CAD build for the part. Positions are in the model's coordinates, mm. A direction names the side the tool comes from. Give positions to 0.01 mm unless a question says otherwise; leave off trailing zeros. Write each loop counter-clockwise with the first axis right and the second up, starting at its lowest first coordinate (ties: lowest second). Pieces come first, ordered by that corner, then holes. Notation, with made-up numbers: (57.5, 22) -> (102.5, 22) arc R25 cw to (102.5, 56) -> close; hole circle Ø7 at (-34.75, 84). An arc over 180 degrees is marked (long way). Answer as a JSON object with one key per item and string values.
```python
from build123d import *

# Parameters (mm, degrees)
F0_W           = 11.5
F0_H           = 30
F1_DEPTH       = 1.5
F2_D           = 2.5
F2_CSINK_D     = 5
F2_CSINK_ANGLE = 90
F4_DEPTH       = 25
F5_R           = 1.49999


# Not quite as in the source:
# - a fillet or chamfer is up to 0.001 mm smaller than in the source, because OpenCascade refuses the exact size


with BuildPart() as f1:
    # F0 (on Front) → F1 (new body)
    with BuildSketch(Plane.XZ):
        with BuildLine():
            ThreePointArc((-3.8116748205, 37.8448306397), (-9.5616748205, 43.5948306397), (-15.3116748205, 37.8448306397))
            Line((-15.3116748205, 37.8448306397), (-3.8116748205, 37.8448306397))
        make_face()
        with Locations((-9.5616748205, 22.8448306397)):
            Rectangle(F0_W, F0_H)
        with BuildLine():
            Line((-3.8116748205, 7.8448306397), (-15.3116748205, 7.8448306397))
            ThreePointArc((-15.3116748205, 7.8448306397), (-9.5616748205, 2.0948306397), (-3.8116748205, 7.8448306397))
        make_face()
    extrude(amount=F1_DEPTH)

    # F2 (through all)
    with Locations(Plane(origin=(0, 0, 0), x_dir=(1, 0, 0), z_dir=(0, 1, 0))):
        with Locations((-9.5616748205, -37.8448306397), (-9.5616748205, -7.8448306397)):
            CounterSinkHole(F2_D / 2, F2_CSINK_D / 2, counter_sink_angle=F2_CSINK_ANGLE)

    # F3 (on face) → F4 (cut)
    with BuildSketch(Plane.XZ):
        with BuildLine():
            Line((-8.1408721001, 19.8448306397), (-8.1408721001, 25.8448306397))
            Line((-8.1408721001, 25.8448306397), (-11.1408721001, 25.8448306397))
            Line((-11.1408721001, 25.8448306397), (-11.1408721001, 19.8448306397))
            ThreePointArc((-11.1408721001, 19.8448306397), (-9.6408721001, 20.3448306397), (-8.1408721001, 19.8448306397))
        make_face()
        with BuildLine():
            ThreePointArc((-7.1408721001, 17.8448306397), (-7.4048041226, 18.9628646284), (-8.1408721001, 19.8448306397))
            Line((-8.1408721001, 19.8448306397), (-8.1408721001, 17.8448306397))
            Line((-8.1408721001, 17.8448306397), (-11.1408721001, 17.8448306397))
            Line((-11.1408721001, 17.8448306397), (-11.1408721001, 19.8448306397))
            ThreePointArc((-11.1408721001, 19.8448306397), (-10.7589060888, 15.6087626622), (-7.1408721001, 17.8448306397))
        make_face()
        with BuildLine():
            Line((-8.1408721001, 17.8448306397), (-8.1408721001, 19.8448306397))
            ThreePointArc((-8.1408721001, 19.8448306397), (-9.6408721001, 20.3448306397), (-11.1408721001, 19.8448306397))
            Line((-11.1408721001, 19.8448306397), (-11.1408721001, 17.8448306397))
            Line((-11.1408721001, 17.8448306397), (-8.1408721001, 17.8448306397))
        make_face()
    extrude(amount=F4_DEPTH, mode=Mode.SUBTRACT)

    # F5 (radius 1.5 in the source; OpenCascade refuses exactly that, so slightly less here)
    f5_edges = [f1.edges().sort_by_distance(p)[0] for p in [
        (-8.140872, -0.75, 25.844831),
        (-11.140872, -0.75, 25.844831),
    ]]
    fillet(f5_edges, radius=F5_R)


solid = f1.part
```
1) Slice it at C-C (x = -6). List the corners of the cut face in (y, z), then the cut area to 3 significant figures.
Model answer:
{"outline": "(-1.5, 3.33) -> (0, 3.33) -> (0, 42.36) -> (-1.5, 42.36) -> close", "area": "58.5 mm2"}
2) Slice it at A-A (y = -0.35). State how many separate pieces and enclosed holes the cut face has, then the cut area to 3 significant figures.
Model answer:
{"separate pieces": "1", "enclosed holes": "3", "area": "384 mm2"}
3) Slice it at B-B (z = 17.5). List the corners of the cut face in (x, y), then the cut area to 3 significant figures.
Model answer:
{"outline": "(-15.31, -1.5) -> (-12.12, -1.5) -> (-12.12, 0) -> (-15.31, 0) -> close; (-7.16, -1.5) -> (-3.81, -1.5) -> (-3.81, 0) -> (-7.16, 0) -> close", "area": "9.82 mm2"}
4) 3-axis set-ups, long thin cutter, end or side, ignore diameter. For faces 4 (the cylindrical face through (-10.69, -0.76, 25.417)), 5 (the flat face through (-12, 0, 23)): which of +Z, -Z, +X, -X, +Y, -Y reach the whole face in a straight line?
Model answer:
{"face 4": "+Y, -Y", "face 5": "+Z, -Z, +X, -X, +Y"}
5) Wall check: probe 1 along X at (y, z) = (-0.55, 24); probe 2 along X at (y, z) = (-0.2, 19.5); probe 3 along X at (y, z) = (-1.15, 4.5). Give the ranges that are in metal, low to high.
Model answer:
{"probe 1": "x = -15.31 to -11.14, -8.14 to -3.81", "probe 2": "x = -15.31 to -11.51, -7.77 to -3.81", "probe 3": "x = -14.24 to -4.88"}
6) Slice it at D-D (z = 5). List the corners of the cut face in (x, y).
Model answer:
{"outline": "(-14.56, -1.5) -> (-4.56, -1.5) -> (-4.56, 0) -> (-14.56, 0) -> close"}
7) Mould opens along Z. For faces 1 (the cylindrical face through (-9.435, -0.74, 43.593)), 2 (the flat face through (-3.812, -1, 23)), 3 (the flat face through (-11.141, -1, 22)) say: released by +Z, released by -Z, zero draft, split by the parting line, or undercut.
Model answer:
{"face 1": "released by +Z", "face 2": "zero draft", "face 3": "undercut"}
